```python
from build123d import *

# Parameters (mm, degrees)
SKETCH_W     = 23
SKETCH_H     = 16
PAD_DEPTH    = 2
SKETCH001_W  = 10
SKETCH001_H  = 2.1
PAD001_DEPTH = 15.75
SKETCH002_W  = 10
SKETCH002_H  = 3
PAD002_DEPTH = 8
SKETCH003_W  = 10
SKETCH003_H  = 3
PAD003_DEPTH = 8
SKETCH004_R  = 1.6
POCKET_DEPTH = 5
SKETCH005_W  = 2
SKETCH005_H  = 4
PAD004_DEPTH = 5.5
FILLET_R     = 2
FILLET001_R  = 4


with BuildPart() as part:
    # Sketch → Pad (new body)
    with BuildSketch(Plane.XY):
        with Locations((11.5, 8)):
            Rectangle(SKETCH_W, SKETCH_H)
    extrude(amount=PAD_DEPTH)

    # Sketch001 (on Face6 of Pad) → Pad001 (join)
    with BuildSketch(Plane.XY.offset(2)):
        with Locations((13, 1.05)):
            Rectangle(SKETCH001_W, SKETCH001_H)
        with Locations((13, 14.95)):
            Rectangle(SKETCH001_W, SKETCH001_H)
    extrude(amount=PAD001_DEPTH)

    # Sketch002 (on Face6 of Pad001) → Pad002 (join)
    with BuildSketch(Plane.XZ):
        with Locations((13, 16.25)):
            Rectangle(SKETCH002_W, SKETCH002_H)
    extrude(amount=PAD002_DEPTH)

    # Sketch003 (on Face15 of Pad002) → Pad003 (join)
    with BuildSketch(Plane(origin=(0, 16, 0), x_dir=(-1, 0, 0), z_dir=(0, 1, 0))):
        with Locations((-13, 16.25)):
            Rectangle(SKETCH003_W, SKETCH003_H)
    extrude(amount=PAD003_DEPTH)

    # Sketch004 (on Face26 of Pad003) → Pocket (cut)
    with BuildSketch(Plane.XY.offset(17.75)):
        with Locations((13, -4)):
            Circle(SKETCH004_R)
        with Locations((13, 20)):
            Circle(SKETCH004_R)
    extrude(amount=-POCKET_DEPTH, mode=Mode.SUBTRACT)

    # Sketch005 → Pad004 (join)
    with BuildSketch(Plane.XY.offset(2)):
        with Locations((4.7, 4)):
            Rectangle(SKETCH005_W, SKETCH005_H)
    extrude(amount=PAD004_DEPTH)

    # Fillet
    fillet_edges = [part.edges().sort_by_distance(p)[0] for p in [
        (13, 16, 14.75),
        (13, 0, 14.75),
    ]]
    fillet(fillet_edges, radius=FILLET_R)

    # Fillet001
    fillet001_edges = [part.edges().sort_by_distance(p)[0] for p in [
        (8, -8, 16.25),
        (18, -8, 16.25),
        (18, 24, 16.25),
        (8, 24, 16.25),
    ]]
    fillet(fillet001_edges, radius=FILLET001_R)


solid = part.part
```
Verification items for the finished model (mm, model axes). A direction names the side the tool comes from. Round coordinates to 2 decimals unless told otherwise and drop trailing zeros. Write each loop counter-clockwise with the first axis right and the second up, starting at its lowest first coordinate (ties: lowest second). Pieces come first, ordered by that corner, then holes.
1. Gauge pin test, flat ends, axial feed: P1, Ø0.6, axis at x = 4.5, z = 4.5, coming from the -Y side; P2, Ø8, axis at x = 11.5, z = 9.5, coming from the +Y side; P3, Ø2, axis at y = 3, z = 5.5, coming from the +X side; P4, Ø1.5, axis at x = 19, z = 5, coming from the -Y side. Record the tip position at first contact, or that the pin passes through.
2. Section check A-A on z = 7. Enter the section's corners in (x, y).
3. Section check D-D on y = -0.5. Enter the section's corners in (x, z), plus the area to 3 significant figures.
4. Access from +Z, -Z, +X, -X, +Y, -Y to the whole of each face (thin tool, end or side, straight path). Record for faces 4 (the flat face through (13, -6, 14.75)), 5 (the flat face through (5, 6, 5)), 6 (the flat face through (5, 2, 5)), 7 (the flat face through (13, 22, 14.75)), 8 (the flat face through (3.7, 4, 5)).
5. Scan lines: L1, parallel to Y at x = 13, z = 15.9; L2, parallel to Y at x = 12.25, z = 2.5; L3, parallel to Z at x = 12.25, y = 10.5. Record each from-to range of solid material in increasing order.
6. Draft check along Y on faces 1 (the flat face through (8, 15.6, 11.5)), 2 (the flat face through (13, 24, 16)), 3 (the flat face through (13, 13.9, 10)). Enter one of: +Y half, -Y half, draft (parallel to the pull), parting line (faces both ways), or undercut.
7. Section check C-C on y = -5. Enter the section's corners in (x, z), plus the area to 3 significant figures.
8. Section check B-B on x = 13. Enter the section's corners in (y, z), plus the area to 3 significant figures.
Answer:
1. P1: stops at y = 2
1. P2: stops at y = 16.15
1. P3: stops at x = 18
1. P4: passes through
2. outline: (3.7, 2) - (5.7, 2) - (5.7, 6) - (3.7, 6) - close; (8, 0) - (18, 0) - (18, 2.1) - (8, 2.1) - close; (8, 13.9) - (18, 13.9) - (18, 16) - (8, 16) - close
3. outline: (8, 14.07) - (18, 14.07) - (18, 17.75) - (8, 17.75) - close
3. area: 36.8 mm2
4. face 4: -Z, +X, -X, -Y
4. face 5: +Z, +X, -X, +Y
4. face 6: +Z, -X, -Y
4. face 7: -Z, +X, -X, +Y
4. face 8: +Z, -X, +Y, -Y
5. L1: y = -8 to -5.6, -2.4 to 2.1, 13.9 to 18.4, 21.6 to 24
5. L2: y = 0 to 2.1, 13.9 to 16
5. L3: z = 0 to 2
6. face 1: draft
6. face 2: +Y half
6. face 3: undercut
7. outline: (8.13, 14.75) - (11.75, 14.75) - (11.75, 17.75) - (8.13, 17.75) - close; (14.25, 14.75) - (17.87, 14.75) - (17.87, 17.75) - (14.25, 17.75) - close
7. area: 21.7 mm2
8. outline: (-8, 14.75) - (-5.6, 14.75) - (-5.6, 17.75) - (-8, 17.75) - close; (-2.4, 14.75) - (-2, 14.75) arc R2 cw to (0, 12.75) - (0, 0) - (16, 0) - (16, 12.75) arc R2 cw to (18, 14.75) - (18.4, 14.75) - (18.4, 17.75) - (13.9, 17.75) - (13.9, 2) - (2.1, 2) - (2.1, 17.75) - (-2.4, 17.75) - close; (21.6, 14.75) - (24, 14.75) - (24, 17.75) - (21.6, 17.75) - close
8. area: 129 mm2
